CAD build for the part. Positions are in the model's coordinates, mm. Face numbers are marked on the shaded views. A direction names the side the tool comes from. Give positions to 0.01 mm unless a question says otherwise; leave off trailing zeros. Loops run counter-clockwise (first coordinate to the right, second up) from the corner with the lowest first, then second, coordinate; pieces in that order, holes last.
Item 1: Saw through at B-B on y = -10.5. Give the cut face in (x, z), plus the area to 3 significant figures.
Item 2: Mould opens along X. For the marked faces 4, 5, 6 and 7 say: released by +X, released by -X, zero draft, split by the parting line, or undercut.
Item 3: Drop flat-ended pins along their axis: P1, Ø3, axis at x = -1, z = 16.5, coming from the -Y side; P2, Ø3, axis at y = -9.26, z = 3.75, coming from the -X side; P3, Ø1.1, axis at x = 6, z = 9.5, coming from the +Y side. Give the stop position or say it passes through.
Item 4: Saw through at A-A on z = 9.5. Give the cut face in (x, y), plus the area to 3 significant figures.
Item 5: Which spindle directions (+Z, -Z, +X, -X, +Y, -Y) get a long thin tool onto all of the face, cutting with end or side? Do the marked faces 1, 2 and 3. Say none if no direction does.
Item 6: Probe probe 1 along X at (y, z) = (5, 3.5); probe 2 along Y at (x, z) = (-0.75, 16); probe 3 along Z at (x, y) = (12.5, 2.5). List the from-to ranges inside material, lowest first.
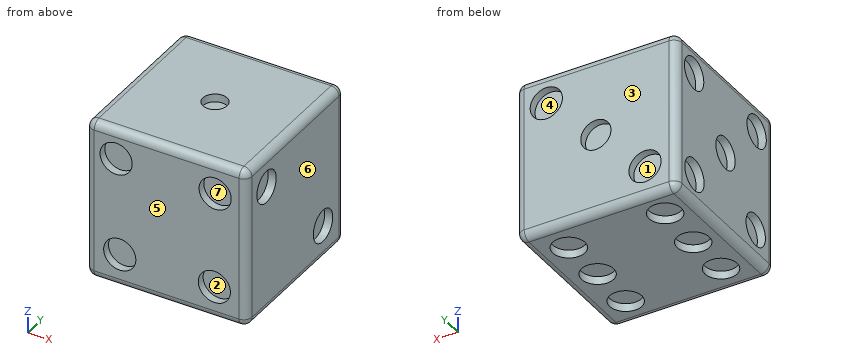
Autodesk Fusion 360 part; units mm, degrees
sketch "Esquisse2" plane through (0, 0, 0) normal (0, 1, 0) x (1, 0, 0)
sketch "Esquisse4" plane through (0, 0, 0) normal (0, 0, 1) x (1, 0, 0)
  line L0 (-4.9636, 6.991) -> (15.0364, 6.991)
  line L1 (15.0364, 6.991) -> (15.0364, -13.009)
  line L2 (15.0364, -13.009) -> (-4.9636, -13.009)
  line L3 (-4.9636, -13.009) -> (-4.9636, 6.991)
  dimension "d9" = 20
  dimension "d10" = 20
extrude "Extrusion1" add sketch "Esquisse4" along normal blind 20
sketch "Esquisse5" plane through (0, 0, 20) normal (0, 0, 1) x (-1, 0, 0)
  line L0 (4.9636, 13.009) -> (-15.0364, 13.009)
  line L1 (-15.0364, 13.009) -> (-15.0364, -6.991)
  line L2 (-15.0364, -6.991) -> (4.9636, -6.991)
  line L3 (4.9636, -6.991) -> (4.9636, 13.009)
  circle A0 centre (-5.0364, 3.009) radius 1.5
  line L4 (-15.0364, 13.009) -> (4.9636, -6.991) construction
  dimension "d15" = 3
extrude "Extrusion2" cut sketch "Esquisse5" against normal blind 1 contours A0
sketch "Esquisse6" plane through (0, 6.991, 0) normal (0, 1, 0) x (-1, 0, 0)
  line L0 (-15.0364, 0) -> (4.9636, 0)
  line L1 (4.9636, 0) -> (4.9636, 20)
  line L2 (4.9636, 20) -> (-15.0364, 20)
  line L3 (-15.0364, 20) -> (-15.0364, 0)
  line L4 (-15.0364, 20) -> (4.9636, 0) construction
  line L5 (4.9636, 20) -> (-15.0364, 0) construction
  circle A0 centre (-5.1366, 10.1002) radius 1.877
  circle A1 centre (0.9787, 3.9849) radius 2
  circle A2 centre (-11.2908, 16.2544) radius 2
  line L6 (-11.2908, 16.2544) -> (-5.1366, 10.1002) construction
  line L7 (-5.1366, 10.1002) -> (0.9787, 3.9849) construction
  dimension "d16" = 4
  dimension "d17" = 4
extrude "Extrusion3" cut sketch "Esquisse6" against normal blind 1 contours A0 | A1 | A2
sketch "Esquisse7" plane through (-4.9636, 0, 0) normal (-1, 0, 0) x (0, -1, 0)
  line L0 (-6.991, 0) -> (13.009, 0)
  line L1 (13.009, 0) -> (13.009, 20)
  line L2 (13.009, 20) -> (-6.991, 20)
  line L3 (-6.991, 20) -> (-6.991, 0)
  line L4 (-6.991, 20) -> (13.009, 0) construction
  line L5 (13.009, 20) -> (-6.991, 0) construction
  circle A0 centre (3.009, 10) radius 2
  circle A1 centre (-3.4749, 16.4839) radius 2
  circle A2 centre (9.2603, 3.7487) radius 2
  circle A3 centre (9.4496, 16.4405) radius 2
  circle A4 centre (-3.4075, 3.5835) radius 2
  dimension "d20" = 4
  dimension "d21" = 4
  dimension "d22" = 4
  dimension "d23" = 4
  dimension "d24" = 4
extrude "Extrusion4" cut sketch "Esquisse7" against normal blind 1 contours A0 | A1 | A2 | A3 | A4
sketch "Esquisse8" plane through (0, 0, 0) normal (0, 0, -1) x (1, 0, 0)
  line L0 (15.0364, 13.009) -> (-4.9636, 13.009)
  line L1 (-4.9636, 13.009) -> (-4.9636, -6.991)
  line L2 (-4.9636, -6.991) -> (15.0364, -6.991)
  line L3 (15.0364, -6.991) -> (15.0364, 13.009)
  line L4 (-4.9636, 13.009) -> (15.0364, -6.991) construction
  line L5 (15.0364, 13.009) -> (-4.9636, -6.991) construction
  circle A0 centre (10.95, -2.9046) radius 2
  circle A1 centre (11.0493, 9.022) radius 2
  circle A2 centre (10.9398, 3.0285) radius 2
  circle A3 centre (-0.8642, 8.9096) radius 2
  circle A4 centre (-1.2323, -3.2596) radius 2
  circle A5 centre (-0.9381, 3.037) radius 2
  dimension "d27" = 4
  dimension "d28" = 4
  dimension "d29" = 4
  dimension "d30" = 4
  dimension "d31" = 4
  dimension "d32" = 4
extrude "Extrusion5" cut sketch "Esquisse8" against normal blind 1 contours A0 | A1 | A2 | A3 | A4 | A5
sketch "Esquisse9" plane through (0, -13.009, 0) normal (0, -1, 0) x (1, 0, 0)
  line L0 (-4.9636, 0) -> (15.0364, 0)
  line L1 (15.0364, 0) -> (15.0364, 20)
  line L2 (15.0364, 20) -> (-4.9636, 20)
  line L3 (-4.9636, 20) -> (-4.9636, 0)
  line L4 (-4.9636, 20) -> (15.0364, 0) construction
  line L5 (15.0364, 20) -> (-4.9636, 0) construction
  circle A0 centre (11.0636, 16.0272) radius 2
  circle A1 centre (10.9669, 4.0694) radius 2
  circle A2 centre (-1.2383, 16.2746) radius 2
  circle A3 centre (-0.7874, 4.1763) radius 2
  dimension "d35" = 4
  dimension "d36" = 4
  dimension "d37" = 4
  dimension "d38" = 4
extrude "Extrusion6" cut sketch "Esquisse9" against normal blind 1 contours A0 | A1 | A2 | A3
sketch "Esquisse10" plane through (15.0364, 0, 0) normal (1, 0, 0) x (0, 1, 0)
  line L0 (-13.009, 0) -> (6.991, 0)
  line L1 (6.991, 0) -> (6.991, 20)
  line L2 (6.991, 20) -> (-13.009, 20)
  line L3 (-13.009, 20) -> (-13.009, 0)
  line L4 (-13.009, 20) -> (6.991, 0) construction
  line L5 (6.991, 20) -> (-13.009, 0) construction
  circle A0 centre (-8.9924, 15.9834) radius 2
  circle A1 centre (2.6774, 4.3136) radius 2
  dimension "d41" = 4
  dimension "d42" = 4
extrude "Extrusion7" cut sketch "Esquisse10" against normal blind 1 contours A0 | A1
fillet "Congé2" radius 1 12 edges at (15.0364, -3.009, 0) (5.0364, -13.009, 0) (-4.9636, -3.009, 0) (5.0364, 6.991, 0) (15.0364, -13.009, 10) (-4.9636, -13.009, 10) (5.0364, -13.009, 20) (15.0364, -3.009, 20) (15.0364, 6.991, 10) (5.0364, 6.991, 20) (-4.9636, 6.991, 10) (-4.9636, -3.009, 20)
fillet "Congé1" [suppressed]
Results below:
1. outline: (-4.96, 1) arc R1 ccw to (-3.96, 0) - (-2.08, 0) - (-2.08, 1) - (0.35, 1) - (0.35, 0) - (9.7, 0) - (9.7, 1) - (12.4, 1) - (12.4, 0) - (14.04, 0) arc R1 ccw to (15.04, 1) - (15.04, 14.67) - (14.04, 14.67) - (14.04, 17.3) - (15.04, 17.3) - (15.04, 19) arc R1 ccw to (14.04, 20) - (-3.96, 20) arc R1 ccw to (-4.96, 19) - (-4.96, 18.14) - (-3.96, 18.14) - (-3.96, 14.74) - (-4.96, 14.74) - (-4.96, 5.32) - (-3.96, 5.32) - (-3.96, 2.18) - (-4.96, 2.18) - close
1. area: 385 mm2
2. face 4: undercut
2. face 5: zero draft
2. face 6: released by +X
2. face 7: undercut
3. P1: stops at y = -12.01
3. P2: stops at x = -3.96
3. P3: stops at y = 5.99
4. outline: (-4.96, -12.01) arc R1 ccw to (-3.96, -13.01) - (14.04, -13.01) arc R1 ccw to (15.04, -12.01) - (15.04, 5.99) arc R1 ccw to (14.04, 6.99) - (6.92, 6.99) - (6.92, 5.99) - (3.36, 5.99) - (3.36, 6.99) - (-3.96, 6.99) arc R1 ccw to (-4.96, 5.99) - (-4.96, -1.07) - (-3.96, -1.07) - (-3.96, -4.95) - (-4.96, -4.95) - close
4. area: 392 mm2
5. face 1: +Y
5. face 2: -Y
5. face 3: +Z, -Z, +X, -X, +Y
6. probe 1: x = -3.96 to 15.04
6. probe 2: y = -12.01 to 6.99
6. probe 3: z = 1 to 20
